from build123d import *

# Parameters (mm, degrees)
BOSS_EXTRUDE1_DEPTH = 35
SKETCH3_R           = 1.4
CUT_EXTRUDE1_DEPTH  = 5
SKETCH4_R           = 1.4
CUT_EXTRUDE2_DEPTH  = 5
CUT_EXTRUDE3_DEPTH  = 2.3
SKETCH6_R           = 0.9
CUT_EXTRUDE4_DEPTH  = 5


with BuildPart() as part:
    # Sketch1 → Boss-Extrude1 (new body)
    with BuildSketch(Plane(origin=(0, 0, 0), x_dir=(1, 0, 0), z_dir=(0, 1, 0))):
        Polygon((0, 0), (5, 0), (40, 0), (40, -5), (40, -25), (35, -25), (35, -5), (5, -5), (5, -80), (0, -80), align=None)
    extrude(amount=BOSS_EXTRUDE1_DEPTH)

    # Sketch3 → Cut-Extrude1 (cut)
    with BuildSketch(Plane(origin=(40, 0, 0), x_dir=(0, 0, -1), z_dir=(1, 0, 0))):
        with Locations((-20, 29)):
            Circle(SKETCH3_R)
        with Locations((-20, 6)):
            Circle(SKETCH3_R)
    extrude(amount=-CUT_EXTRUDE1_DEPTH, mode=Mode.SUBTRACT)

    # Sketch4 → Cut-Extrude2 (cut)
    with BuildSketch(Plane.ZY):
        with Locations((10, 29.3)):
            Circle(SKETCH4_R)
        with Locations((57.6, 29.3)):
            Circle(SKETCH4_R)
        with Locations((57.6, 5.7)):
            Circle(SKETCH4_R)
        with Locations((10, 5.7)):
            Circle(SKETCH4_R)
    extrude(amount=-CUT_EXTRUDE2_DEPTH, mode=Mode.SUBTRACT)

    # Sketch5 → Cut-Extrude3 (cut)
    with BuildSketch(Plane.ZY):
        Polygon((1.305296416, 33.993673453), (0.792101755, 32.895205775), (1.486805338, 31.901532322), (2.694703584, 32.006326547), (3.207898245, 33.104794225), (2.513194662, 34.098467678), align=None)
        Polygon((2.614505204, 3.045171447), (1.402107578, 3.054762841), (0.787602373, 2.009591394), (1.385494796, 0.954828553), (2.597892422, 0.945237159), (3.212397627, 1.990408606), align=None)
        Polygon((78.957273376, 2.744061612), (77.83426043, 3.201053868), (76.876987054, 2.456992256), (77.042726624, 1.255938388), (78.16573957, 0.798946132), (79.123012946, 1.543007744), align=None)
        Polygon((78.740718882, 33.959862249), (77.539094349, 34.121412494), (76.798375467, 33.161550244), (77.259281118, 32.040137751), (78.460905651, 31.878587506), (79.201624533, 32.838449756), align=None)
    extrude(amount=-CUT_EXTRUDE3_DEPTH, mode=Mode.SUBTRACT)

    # Sketch6 → Cut-Extrude4 (cut)
    with BuildSketch(Plane.ZY):
        with Locations((77, 25.5)):
            Circle(SKETCH6_R)
        with Locations((77, 9.5)):
            Circle(SKETCH6_R)
    extrude(amount=-CUT_EXTRUDE4_DEPTH, mode=Mode.SUBTRACT)


solid = part.part
Build history of the part. All positions in model axes, mm. A direction names the side the tool comes from. Give positions to 0.01 mm unless a question says otherwise; leave off trailing zeros. Order: outer loops, then holes, each group sorted by start corner. A loop starts at its lowest first (then second) coordinate and runs counter-clockwise, first axis right, second up. Notation, with made-up numbers: M 43.5,89.25 L 94.5,89.25 A29 ccw 94.5,126.25 Z; hole C 44,76 d10. An arc over 180 degrees is marked long. Put each result on its own line as item: value.
Item 1: Cut at A-A on z = 57.6. Write the cut outline in (x, y).
Results are:
outline: M 0,0 L 5,0 L 5,4.3 L 0,4.3 Z; M 0,7.1 L 5,7.1 L 5,27.9 L 0,27.9 Z; M 0,30.7 L 5,30.7 L 5,35 L 0,35 Z
Item 2: Cut at C-C on y = 9.5. Write the cut outline in (x, z), then the cut area to 3 significant figures.
Results are:
outline: M 0,0 L 40,0 L 40,25 L 35,25 L 35,5 L 5,5 L 5,76.1 L 0,76.1 Z; M 0,77.9 L 5,77.9 L 5,80 L 0,80 Z
area: 666 mm2
Item 3: Wall check: probe 1 along Y at (x, z) = (37.8, 20); probe 2 along Y at (x, z) = (2, 57); probe 3 along Z at (x, y) = (3, 5). Give the ranges that are in metal, low to high.
Results are:
probe 1: 0 to 4.6, 7.4 to 27.6, 30.4 to 35
probe 2: 0 to 4.44, 6.96 to 28.04, 30.56 to 35
probe 3: 0 to 8.79, 11.21 to 56.39, 58.81 to 80
Item 4: Drop flat-ended pins along their axis: pin 1 Ø10 at (x, y) = (18, 13) entering from +Z; pin 2 Ø2.5 at (y, z) = (9.5, 77) entering from +X; pin 3 Ø4 at (x, y) = (38.5, 11) entering from +Z. Give the stop position or say it passes through.
Results are:
pin 1: z = 5
pin 2: x = 5
pin 3: z = 25
Item 5: Cut at D-D on x = 32.5. Write the cut outline in (y, z).
Results are:
outline: M 0,0 L 35,0 L 35,5 L 0,5 Z
Item 6: Cut at B-B on z = 20. Write the cut outline in (x, y), then the cut area to 3 significant figures.
Results are:
outline: M 0,0 L 5,0 L 5,35 L 0,35 Z; M 35,0 L 40,0 L 40,4.6 L 35,4.6 Z; M 35,7.4 L 40,7.4 L 40,27.6 L 35,27.6 Z; M 35,30.4 L 40,30.4 L 40,35 L 35,35 Z
area: 322 mm2
Item 7: Which spindle directions (+Z, -Z, +X, -X, +Y, -Y) get a long thin tool onto all of the face, cutting with end or side? Do faces 1 (the face through (37.53, 30.39, 20.18)), 2 (the face through (20, 17, 5)), 3 (the face through (2.3, 2, 2)). Say none if no direction does.
Results are:
face 1: +X
face 2: +Z, +Y, -Y
face 3: -X
Item 8: Pull direction Z, two halves, no side cores. Call faces 4 (the face through (38, 17, 25)), 5 (the face through (5, 17, 42)), 6 (the face through (2.46, 28.45, 8.89)): +Z half, -Z half, draft (parallel to the pull), parting line (faces both ways), or undercut.
Results are:
face 4: +Z half
face 5: draft
face 6: undercut
